```python
from build123d import *

# Parameters (mm, degrees)
BOSS_EXTRUDE1_DEPTH = 2.65684
SKETCH2_R           = 38.1
CUT_EXTRUDE1_DEPTH  = 3.65684
SKETCH3_R           = 6.35
CUT_EXTRUDE2_DEPTH  = 3.65684


with BuildPart() as part:
    # Sketch1 → Boss-Extrude1 (new body)
    with BuildSketch(Plane(origin=(0, 0, 0), x_dir=(1, 0, 0), z_dir=(0, 1, 0))):
        Polygon((0, 450.85), (0, 0), (546.1, 0), (546.1, 25.4), align=None)
    extrude(amount=BOSS_EXTRUDE1_DEPTH)

    # Sketch2 → Cut-Extrude1 (cut, through all)
    with BuildSketch(Plane.XZ):
        with Locations((254, -114.3)):
            Circle(SKETCH2_R)
    extrude(amount=-CUT_EXTRUDE1_DEPTH, mode=Mode.SUBTRACT)

    # Sketch3 → Cut-Extrude2 (cut, through all)
    with BuildSketch(Plane(origin=(0, 2.65684, 0), x_dir=(1, 0, 0), z_dir=(0, 1, 0))):
        with Locations((362.072773191, 77.087559946)):
            Circle(SKETCH3_R)
        with Locations((167.736694981, 39.312452986)):
            Circle(SKETCH3_R)
        with Locations((232.190531828, 226.499987068)):
            Circle(SKETCH3_R)
    extrude(amount=-CUT_EXTRUDE2_DEPTH, mode=Mode.SUBTRACT)


solid = part.part
```
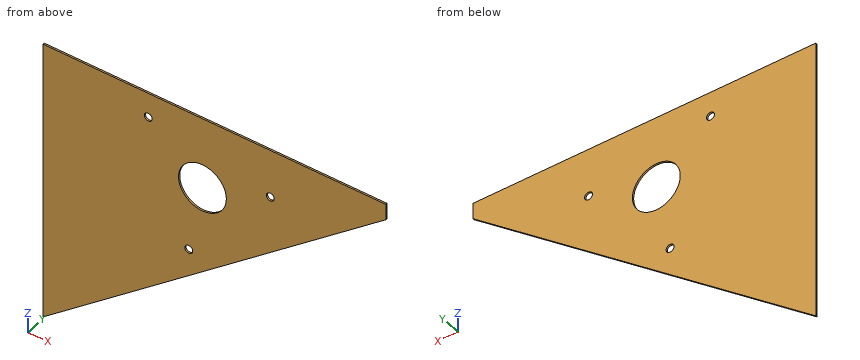
Source: CAD feature listing. Evaluate the final solid. Frame: model axes, mm. Coordinates: 2 decimals unless noted, no trailing zeros. Loops run counter-clockwise (first coordinate to the right, second up) from the corner with the lowest first, then second, coordinate; pieces in that order, holes last. Notation, with made-up numbers: (68, 31) - (113, 31) arc R14 ccw to (113, 45) - close; hole circle Ø7 at (83, 0.5). An arc over 180 degrees is marked (long way). Answer as CSV lines item,"result".
1. Section D-D (x = 122). Return loops of the section in (y, z).
Established:
outline,"(0, -355.8) - (2.66, -355.8) - (2.66, 0) - (0, 0) - close"
2. Ray query, line 1 (Z direction, x = 231.5, y = 1.8); line 2 (X direction, y = 1.3, z = -224); line 3 (X direction, y = 1.75, z = -73). Return the intervals inside material, ascending.
Established:
line 1,"z = -270.5 to -232.81, -220.19 to -145.05, -83.55 to 0"
line 2,"x = 0 to 226.35, 238.03 to 291.18"
line 3,"x = 0 to 357.21, 366.93 to 485"
3. Section C-C (y = 0.45). Return loops of the section in (x, z), then the cut area to 3 significant figures.
Established:
outline,"(0, -450.85) - (546.1, -25.4) - (546.1, 0) - (0, 0) - close; hole circle Ø12.7 at (167.74, -39.31); hole circle Ø76.2 at (254, -114.3); hole circle Ø12.7 at (232.19, -226.5); hole circle Ø12.7 at (362.07, -77.09)"
area,"125,000 mm2"
4. Contact query for flat-ended pins moving along their axis: pin 1 (10 mm diameter, centred on x = 167.74, z = -39.31, fed in from -Y); pin 2 (14.5 mm diameter, centred on x = 232.19, z = -226.5, fed in from +Y); pin 3 (1 mm diameter, centred on x = 299, y = 1, fed in from -Z). Output: stop coordinate, or through.
Established:
pin 1,"passes through"
pin 2,"stops at y = 2.66"
pin 3,"stops at z = -218.3"
5. Section B-B (z = -114.3). Return loops of the section in (x, y).
Established:
outline,"(0, 0) - (215.9, 0) - (215.9, 2.66) - (0, 2.66) - close; (292.1, 0) - (431.99, 0) - (431.99, 2.66) - (292.1, 2.66) - close"
6. Section A-A (x = 254). Return loops of the section in (y, z), then the cut area to 3 significant figures.
Established:
outline,"(0, -252.97) - (2.66, -252.97) - (2.66, -152.4) - (0, -152.4) - close; (0, -76.2) - (2.66, -76.2) - (2.66, 0) - (0, 0) - close"
area,"470 mm2"
